Source: three-view drawing plus pictorial views. Frame: mm from the lowest corner of the part. Round coordinates to 2 decimals unless told otherwise and drop trailing zeros. Answer as a JSON object with one key per item and string values. Group by question number.
Item 1: Section query C-C on x = 83.5. Count the separate pieces of the cut face and the enclosed holes in it.
Item 2: Pin query (flat end, axial travel): pin 1 (7.5 mm diameter, centred on x = 35.1, z = 85.1, fed in from +Y) (3 decimals); pin 2 (4 mm diameter, centred on x = 54.5, z = 89, fed in from +Y); pin 3 (7.5 mm diameter, centred on x = 85.1, z = 85.1, fed in from -Y); pin 4 (1.5 mm diameter, centred on y = 2.5, z = 48.5, fed in from -X). Return the tip coordinate at first contact, or that it passes through.
Item 3: Material intervals for line 1 (X direction, y = 4.5, z = 35.1) (1 decimal); line 2 (X direction, y = 4.75, z = 84.5) (1 decimal); line 3 (Z direction, x = 36, y = 3.5) (1 decimal), sorted ascending. Write a range as [from, to].
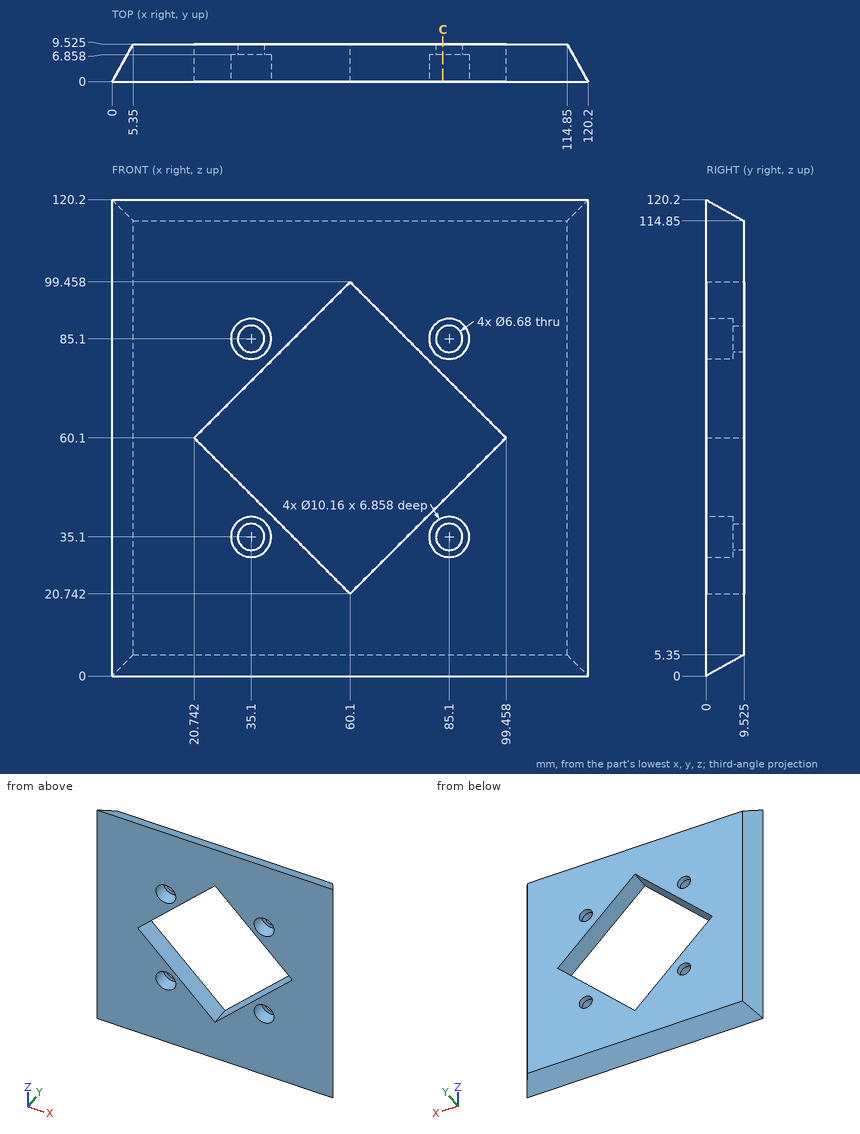
Solved:
{
 "1": {"separate pieces": "4", "enclosed holes": "0"},
 "2": {"pin 1": "y = 9.525", "pin 2": "through", "pin 3": "y = 6.86", "pin 4": "x = 0.98"},
 "3": {"line 1": "[2.5, 30], [40.2, 45.7], [74.5, 80], [90.2, 117.7]", "line 2": "[2.7, 30.1], [40.1, 45.1], [75.1, 80.1], [90.1, 117.5]", "line 3": "[2, 30.1], [40.1, 44.8], [75.4, 80.1], [90.1, 118.2]"}
}
